from build123d import *

# Parameters (mm, degrees)
SKETCH1_W                    = 100
SKETCH1_H                    = 45
BASE_FLANGE1_DEPTH           = 3
EDGE_FLANGE1_STRIP_W         = 14
EDGE_FLANGE1_STRIP_H         = 3
EDGE_FLANGE1_STRIP_CUT_DEPTH = 100
EDGE_FLANGE1_DEPTH           = 100
EDGE_FLANGE2_STRIP_W         = 14
EDGE_FLANGE2_STRIP_H         = 3
EDGE_FLANGE2_STRIP_CUT_DEPTH = 100
EDGE_FLANGE2_DEPTH           = 100
SKETCH12_R                   = 2
CUT_EXTRUDE1_DEPTH           = 64.144675152
F_4_0MM_DOWEL_HOLE1_D        = 4
F_4_0MM_DOWEL_HOLE1_DEPTH    = 12.4
F_4_0MM_DOWEL_HOLE1_TIP      = 1.201721238
CHAMFER1_SIZE                = 30


# Sheet-metal steps are written as plain solids
with BuildPart() as part:
    # Sketch1 → Base-Flange1 (new body)
    with BuildSketch(Plane(origin=(0, 0, 0), x_dir=(1, 0, 0), z_dir=(0, 1, 0))):
        Rectangle(SKETCH1_W, SKETCH1_H)
    extrude(amount=-BASE_FLANGE1_DEPTH)

    # Edge-Flange1 strip (across the edge) → Edge-Flange1 strip cut (cut)
    with BuildSketch(Plane(origin=(-50, -3, -22.5), x_dir=(0, 0, 1), z_dir=(1, 0, 0))):
        with Locations((-3, -1.5)):
            Rectangle(EDGE_FLANGE1_STRIP_W, EDGE_FLANGE1_STRIP_H)
    extrude(amount=EDGE_FLANGE1_STRIP_CUT_DEPTH, mode=Mode.SUBTRACT)

    # Edge-Flange1 section (across the edge) → Edge-Flange1 (add)
    with BuildSketch(Plane(origin=(-50, -3, -22.5), x_dir=(0, 0, 1), z_dir=(1, 0, 0))):
        with BuildLine():
            Line((0, 1), (0, 9))
            Line((0, 9), (3, 9))
            Line((3, 9), (3, 1))
            ThreePointArc((3, 1), (3.292893219, 0.292893219), (4, 0))
            Line((4, 0), (4, -3))
            ThreePointArc((4, -3), (1.171572875, -1.828427125), (0, 1))
        make_face()
    extrude(amount=EDGE_FLANGE1_DEPTH)

    # Edge-Flange2 strip (across the edge) → Edge-Flange2 strip cut (cut)
    with BuildSketch(Plane(origin=(50, -12, -22.5), x_dir=(0, 1, 0), z_dir=(-1, 0, 0))):
        with Locations((-3, -1.5)):
            Rectangle(EDGE_FLANGE2_STRIP_W, EDGE_FLANGE2_STRIP_H)
    extrude(amount=EDGE_FLANGE2_STRIP_CUT_DEPTH, mode=Mode.SUBTRACT)

    # Edge-Flange2 section (across the edge) → Edge-Flange2 (add)
    with BuildSketch(Plane(origin=(50, -12, -22.5), x_dir=(0, 1, 0), z_dir=(-1, 0, 0))):
        with BuildLine():
            Line((0, 1), (0, 15))
            Line((0, 15), (3, 15))
            Line((3, 15), (3, 1))
            ThreePointArc((3, 1), (3.292893219, 0.292893219), (4, 0))
            Line((4, 0), (4, -3))
            ThreePointArc((4, -3), (1.171572875, -1.828427125), (0, 1))
        make_face()
    extrude(amount=EDGE_FLANGE2_DEPTH)

    # Sketch12 → Cut-Extrude1 (cut, through all)
    with BuildSketch(Plane(origin=(0, -9, 0), x_dir=(1, 0, 0), z_dir=(0, 1, 0))):
        with Locations(Location((-27.5, 32.5, 0), (0, 0, 270))):
            Circle(SKETCH12_R)
        with Locations(Location((27.5, 32.5, 0), (0, 0, 270))):
            Circle(SKETCH12_R)
    extrude(amount=-CUT_EXTRUDE1_DEPTH, mode=Mode.SUBTRACT)

    # Ø4.0mm Dowel Hole1
    with Locations(Plane(origin=(12, 0, -15), x_dir=(0, 0, 1), z_dir=(0, 1, 0))):
        with Locations((0, 0), (30, 0), (30, -24), (0, -24)):
            Hole(F_4_0MM_DOWEL_HOLE1_D / 2, depth=F_4_0MM_DOWEL_HOLE1_DEPTH)
            with Locations((0, 0, -(F_4_0MM_DOWEL_HOLE1_DEPTH + F_4_0MM_DOWEL_HOLE1_TIP / 2))):  # 118° drill point
                Cone(0, F_4_0MM_DOWEL_HOLE1_D / 2, F_4_0MM_DOWEL_HOLE1_TIP, mode=Mode.SUBTRACT)

    # Chamfer1
    chamfer1_edges = [part.edges().sort_by_distance(p)[0] for p in [
        (50, -1.5, 22.5),
        (-50, -1.5, 22.5),
    ]]
    chamfer(chamfer1_edges, length=CHAMFER1_SIZE)


solid = part.part
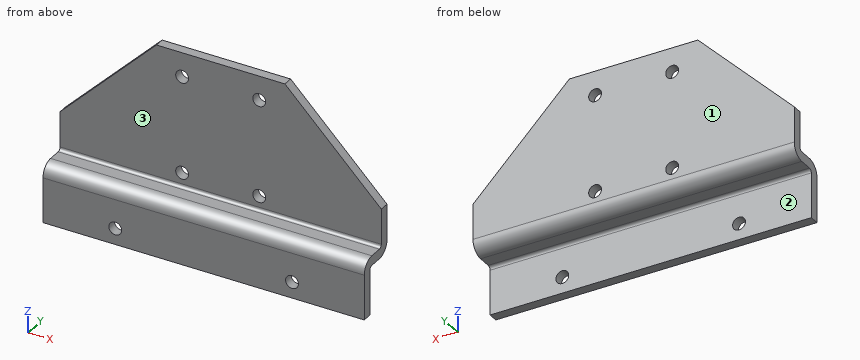
Can you work these out from the model? Positions are in its coordinate system, mm. Face numbers are marked on the shaded views. A direction names the side the tool comes from. Give positions to 0.01 mm unless a question says otherwise; leave off trailing zeros. Write each loop counter-clockwise with the first axis right and the second up, starting at its lowest first coordinate (ties: lowest second). Pieces come first, ordered by that corner, then holes. Notation, with made-up numbers: (-29, -10.5) -> (-6, -10.5) arc R20 cw to (-6, 21.5) -> close; hole circle Ø7 at (-35.75, 57). An arc over 180 degrees is marked (long way). Answer as a JSON object with one key per item and string values. Group by question number.
Item 1: Please list where these lines run through material, in increasing order: line 1 (X direction, y = -10.35, z = -32.5); line 2 (X direction, y = -0.85, z = -15); line 3 (Y direction, x = -31.5, z = -31.5). Write a range as [from, to].
Item 2: Suppose I cut it at D-D (y = -1.5). Please give me the cut outline in (x, z).
Item 3: I'm going to push flat-ended pins straight in: P1, Ø20.5, axis at x = 13, z = 8.5, coming from the -Y side; P2, Ø5, axis at x = 12.5, z = -20, coming from the -Y side; P3, Ø4.5, axis at x = -27.5, z = -32.5, coming from the +Y side. Where does each tip first touch, or does it pass through?
Item 4: For the marked faces 1, 2 and 3, which set-ups out of +Z, -Z, +X, -X, +Y, -Y let a thin tool reach every point of the face, with its end or its side?
Item 5: Suppose I cut it at B-B (z = 15). Please give me the cut outline in (x, y), plus the area to 3 significant figures.
Item 6: Suppose I cut it at C-C (x = -12). Please give me the cut outline in (y, z), plus the area to 3 significant figures.
Item 7: Suppose I cut it at A-A (x = -27.5). Please give me the cut outline in (y, z).
Findings:
{
 "1": {"line 1": "x = [-50, -29.5], [-25.5, 25.5], [29.5, 50]", "line 2": "x = [-50, -14], [-10, 10], [14, 50]", "line 3": "y = [-12, -9]"},
 "2": {"outline": "(-50, -21.62) -> (50, -21.62) -> (50, -7.5) -> (20, 22.5) -> (-20, 22.5) -> (-50, -7.5) -> close; hole circle Ø4 at (-12, -15); hole circle Ø4 at (-12, 15); hole circle Ø4 at (12, -15); hole circle Ø4 at (12, 15)"},
 "3": {"P1": "stops at y = -3", "P2": "stops at y = -11.87", "P3": "stops at y = -9"},
 "4": {"face 1": "+Z, -Z, +X, -X, +Y", "face 2": "-Z, +X, -X, +Y", "face 3": "+Z, +X, -X, -Y"},
 "5": {"outline": "(-27.5, -3) -> (-14, -3) -> (-14, 0) -> (-27.5, 0) -> close; (-10, -3) -> (10, -3) -> (10, 0) -> (-10, 0) -> close; (14, -3) -> (27.5, -3) -> (27.5, 0) -> (14, 0) -> close", "area": "141 mm²"},
 "6": {"outline": "(-12, -37.5) -> (-9, -37.5) -> (-9, -23.5) arc R1 cw to (-8, -22.5) -> (-4, -22.5) arc R4 ccw to (0, -18.5) -> (0, -17) -> (-3, -17) -> (-3, -18.5) arc R1 cw to (-4, -19.5) -> (-8, -19.5) arc R4 ccw to (-12, -23.5) -> close; (-3, -13) -> (0, -13) -> (0, 13) -> (-3, 13) -> close; (-3, 17) -> (0, 17) -> (0, 22.5) -> (-3, 22.5) -> close", "area": "177 mm²"},
 "7": {"outline": "(-12, -37.5) -> (-9, -37.5) -> (-9, -34.5) -> (-12, -34.5) -> close; (-12, -30.5) -> (-9, -30.5) -> (-9, -23.5) arc R1 cw to (-8, -22.5) -> (-4, -22.5) arc R4 ccw to (0, -18.5) -> (0, 15) -> (-3, 15) -> (-3, -18.5) arc R1 cw to (-4, -19.5) -> (-8, -19.5) arc R4 ccw to (-12, -23.5) -> close"}
}
